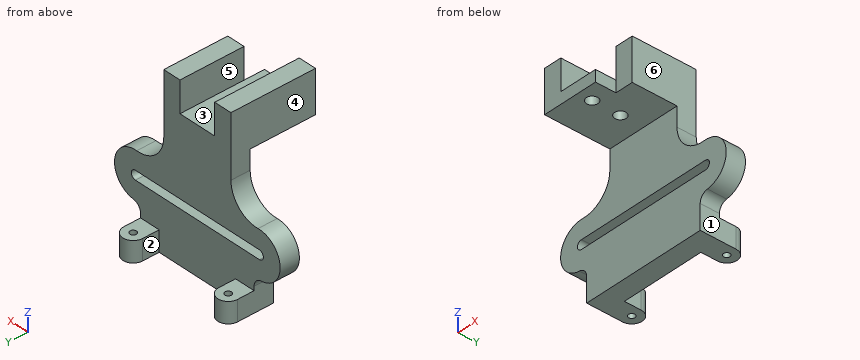
from build123d import *

# Parameters (mm, degrees)
BOSS_EXTRUDE1_DEPTH     = 15
SKETCH2_R               = 2.5
BOSS_EXTRUDE2_DEPTH     = 16
BOSS_EXTRUDE3_DEPTH     = 51
CUT_EXTRUDE1_DEPTH      = 140.202191075
CUT_EXTRUDE1_DEPTH_BACK = 140.202191075
SKETCH4_R               = 4.5
SKETCH4_W               = 14
SKETCH4_H               = 16


with BuildPart() as part:
    # Sketch1 → Boss-Extrude1 (new body)
    with BuildSketch(Plane(origin=(0, 0, 0), x_dir=(1, 0, 0), z_dir=(0, 1, 0))):
        with BuildLine():
            Line((49, 0), (-49, 0))
            Line((-49, 0), (-49, -19.125314072))
            ThreePointArc((-49, -19.125314072), (-50.808661059, -23.821056825), (-55.3, -26.090226132))
            ThreePointArc((-55.3, -26.090226132), (-71.440466452, -45.462758858), (-52.375, -61.964809351))
            ThreePointArc((-52.375, -61.964809351), (-35.937629669, -67.886680846), (-29, -83.921798557))
            Line((-29, -83.921798557), (-29, -132))
            Line((-29, -132), (-15, -132))
            Line((-15, -132), (-15, -108))
            Line((-15, -108), (15, -108))
            Line((15, -108), (15, -132))
            Line((15, -132), (29, -132))
            Line((29, -132), (29, -83.921798557))
            ThreePointArc((29, -83.921798557), (35.937629669, -67.886680846), (52.375, -61.964809351))
            ThreePointArc((52.375, -61.964809351), (71.440466452, -45.462758858), (55.3, -26.090226132))
            ThreePointArc((55.3, -26.090226132), (50.808661059, -23.821056825), (49, -19.125314072))
            Line((49, -19.125314072), (49, 0))
        make_face()
        with BuildLine():
            Line((-53.5, -40.5), (53.5, -40.5))
            ThreePointArc((53.5, -40.5), (57, -44), (53.5, -47.5))
            Line((53.5, -47.5), (-53.5, -47.5))
            ThreePointArc((-53.5, -47.5), (-57, -44), (-53.5, -40.5))
        make_face(mode=Mode.SUBTRACT)
    extrude(amount=BOSS_EXTRUDE1_DEPTH)

    # Sketch2 → Boss-Extrude2 (add)
    # profile 1 of 2: a face of its own
    with BuildSketch(Plane.XY):
        with BuildLine():
            Line((-49, 15), (-49, 28))
            ThreePointArc((-49, 28), (-41, 36), (-33, 28))
            Line((-33, 28), (-33, 15))
            Line((-33, 15), (-49, 15))
        make_face()
        with Locations((-41, 28)):
            Circle(SKETCH2_R, mode=Mode.SUBTRACT)
    # profile 2 of 2: a face of its own
    with BuildSketch(Plane.XY):
        with BuildLine():
            Line((33, 15), (49, 15))
            Line((49, 15), (49, 28))
            ThreePointArc((49, 28), (41, 36), (33, 28))
            Line((33, 28), (33, 15))
        make_face()
        with Locations(Location((41, 28, 0), (0, 0, 180))):
            Circle(SKETCH2_R, mode=Mode.SUBTRACT)
    extrude(amount=BOSS_EXTRUDE2_DEPTH)

    # Sketch3 → Boss-Extrude3 (add)
    with BuildSketch(Plane.XZ):
        Polygon((-15, 108), (15, 108), (15, 132), (29, 132), (29, 99), (-29, 99), (-29, 132), (-15, 132), align=None)
    extrude(amount=BOSS_EXTRUDE3_DEPTH)

    # Sketch4 → Cut-Extrude1 (cut, two sides: drawn at the far end of the back side and taken through both)
    with BuildSketch(Plane.XY.offset(108).offset(-CUT_EXTRUDE1_DEPTH_BACK)):
        with Locations((0, -18)):
            Circle(SKETCH4_R)
        with Locations((0, -40)):
            Circle(SKETCH4_R)
        with Locations((22, -43)):
            Rectangle(SKETCH4_W, SKETCH4_H)
    extrude(amount=CUT_EXTRUDE1_DEPTH + CUT_EXTRUDE1_DEPTH_BACK, mode=Mode.SUBTRACT)


solid = part.part
Check sheet for the modelled part. Datum: model origin and axes. Units: mm. Face numbers are marked on the shaded views. A direction names the side the tool comes from. Coordinates: 2 decimals unless noted, no trailing zeros. Loops run counter-clockwise (first coordinate to the right, second up) from the corner with the lowest first, then second, coordinate; pieces in that order, holes last. Notation, with made-up numbers: (71, 60.5) -> (119, 60.5) arc R24 ccw to (119, 72.5) -> close; hole circle Ø7 at (73, 10.5). An arc over 180 degrees is marked (long way). Write item = value, one per line. Start each with the question number.
1. Section check B-B on y = -18. Record the cut outline in (x, z), then the cut area to 3 significant figures.
2. Section check C-C on x = 0. Record the cut outline in (y, z).
3. Section check D-D on z = 110. Record the cut outline in (x, y).
4. Draft check along X on the marked faces 4, 5 and 6. Enter one of: released by +X, released by -X, zero draft, split by the parting line, or undercut.
5. Depth check by flat-ended pin: P1, Ø5, axis at x = -40.5, y = 30, coming from the +Z side; P2, Ø14.5, axis at y = -19, z = 116.5, coming from the -X side; P3, Ø2, axis at x = -28.5, z = 59, coming from the +Y side; P4, Ø16.5, axis at x = 4, y = 5, coming from the -Z side. Enter the tip coordinate at first touch or a pass-through.
6. Section check A-A on x = 24.5. Record the cut outline in (y, z).
7. Material ranges on line 1 (Y direction, x = 0, z = 102); line 2 (X direction, y = 11.5, z = 116.5); line 3 (X direction, y = -40, z = 104.75), recorded low to high.
8. Tool access check on the marked faces 1, 2 and 3. Record the directions out of +Z, -Z, +X, -X, +Y, -Y that give a thin tool (end or side, any length) a straight path to the whole face; none if there is none.
Responses:
q1.outline = (-29, 99) -> (-4.5, 99) -> (-4.5, 108) -> (-15, 108) -> (-15, 132) -> (-29, 132) -> close; (4.5, 99) -> (29, 99) -> (29, 132) -> (15, 132) -> (15, 108) -> (4.5, 108) -> close
q1.area = 1,110 mm2
q2.outline = (-51, 99) -> (-44.5, 99) -> (-44.5, 108) -> (-51, 108) -> close; (-35.5, 99) -> (-22.5, 99) -> (-22.5, 108) -> (-35.5, 108) -> close; (-13.5, 99) -> (0, 99) -> (0, 47.5) -> (15, 47.5) -> (15, 108) -> (-13.5, 108) -> close; (0, 0) -> (15, 0) -> (15, 40.5) -> (0, 40.5) -> close
q3.outline = (-29, -51) -> (-15, -51) -> (-15, 15) -> (-29, 15) -> close; (15, -35) -> (29, -35) -> (29, 15) -> (15, 15) -> close
q4.face_4 = released by -X
q4.face_5 = undercut
q4.face_6 = released by +X
q5.P1 = 16
q5.P2 = -29
q5.P3 = 15
q5.P4 = 0
q6.outline = (-35, 99) -> (0, 99) -> (0, 47.5) -> (15, 47.5) -> (15, 132) -> (-35, 132) -> close; (0, 0) -> (15, 0) -> (15, 40.5) -> (0, 40.5) -> close
q7.line_1 = -51 to -44.5, -35.5 to -22.5, -13.5 to 15
q7.line_2 = -29 to -15, 15 to 29
q7.line_3 = -29 to -4.5, 4.5 to 15
q8.face_1 = -Z, +X, +Y, -Y
q8.face_2 = +Z, -Z, +Y
q8.face_3 = +Z, +Y, -Y
